Verification items for the finished model (mm, model axes). Face numbers are marked on the shaded views. Coordinates: 2 decimals unless noted, no trailing zeros. Use one line per item in the form item = value. Start each with the question number.
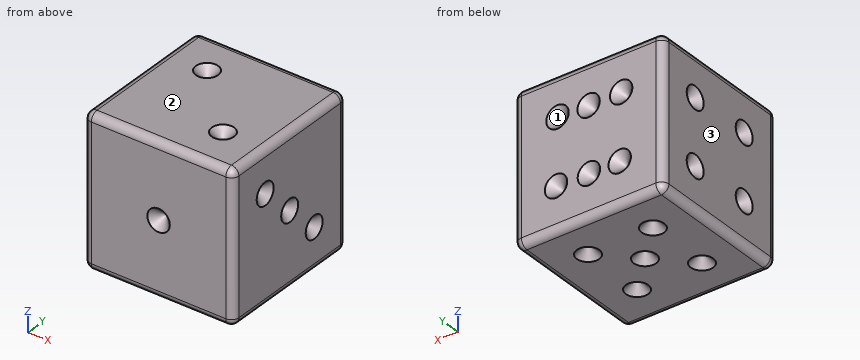
```python
from build123d import *

# Parameters (mm, degrees)
F0_W      = 20
F0_H      = 20
F1_DEPTH  = 20
F2_R      = 1.5
F3_DEPTH  = 1.5
F4_R      = 1
F5_R      = 1.5
F6_DEPTH  = 1.5
F7_R      = 1.5
F8_DEPTH  = 1.5
F9_R      = 1.5
F10_DEPTH = 1.5
F11_R     = 1.5
F12_DEPTH = 1.5
F13_R     = 1.5
F14_DEPTH = 1.5
F15_SIZE  = 1.49999


# Not quite as in the source:
# - a fillet or chamfer is up to 0.001 mm smaller than in the source, because OpenCascade refuses the exact size


with BuildPart() as f1:
    # F0 (on Top) → F1 (new body)
    with BuildSketch(Plane.XY):
        with Locations((10, 10)):
            Rectangle(F0_W, F0_H)
    extrude(amount=F1_DEPTH)

    # F2 (on face) → F3 (cut)
    with BuildSketch(Plane.XZ):
        with Locations((10, 10)):
            Circle(F2_R)
    extrude(amount=-F3_DEPTH, mode=Mode.SUBTRACT)

    # F4
    f4_edges = [f1.edges().sort_by_distance(p)[0] for p in [
        (10, 0, 20),
        (20, 10, 20),
        (20, 0, 10),
        (0, 0, 10),
        (10, 0, 0),
        (20, 10, 0),
        (0, 10, 20),
        (10, 20, 20),
        (0, 10, 0),
        (0, 20, 10),
        (20, 20, 10),
        (10, 20, 0),
    ]]
    fillet(f4_edges, radius=F4_R)

    # F5 (on face) → F6 (cut)
    with BuildSketch(Plane.XY.offset(20)):
        with Locations((5.6568542495, 14.3431457505)):
            Circle(F5_R)
        with Locations((14.3431457505, 5.6568542495)):
            Circle(F5_R)
    extrude(amount=-F6_DEPTH, mode=Mode.SUBTRACT)

    # F7 (on face) → F8 (cut)
    with BuildSketch(Plane.YZ.offset(20)):
        with Locations((5.6568542495, 14.3431457505)):
            Circle(F7_R)
        with Locations((10, 10)):
            Circle(F7_R)
        with Locations((14.3431457505, 5.6568542495)):
            Circle(F7_R)
    extrude(amount=-F8_DEPTH, mode=Mode.SUBTRACT)

    # F9 (on face) → F10 (cut)
    with BuildSketch(Plane(origin=(0, 0, 0), x_dir=(0, -1, 0), z_dir=(-1, 0, 0))):
        with Locations((-14.3431457505, 14.3431457505)):
            Circle(F9_R)
        with Locations((-5.6568542495, 14.3431457505)):
            Circle(F9_R)
        with Locations((-14.3431457505, 5.6568542495)):
            Circle(F9_R)
        with Locations((-5.6568542495, 5.6568542495)):
            Circle(F9_R)
    extrude(amount=-F10_DEPTH, mode=Mode.SUBTRACT)

    # F11 (on face) → F12 (cut)
    with BuildSketch(Plane(origin=(0, 0, 0), x_dir=(1, 0, 0), z_dir=(0, 0, -1))):
        with Locations((5.6568542495, -5.6568542495)):
            Circle(F11_R)
        with Locations((10, -10)):
            Circle(F11_R)
        with Locations((14.3431457505, -5.6568542495)):
            Circle(F11_R)
        with Locations((5.6568542495, -14.3431457505)):
            Circle(F11_R)
        with Locations((14.3431457505, -14.3431457505)):
            Circle(F11_R)
    extrude(amount=-F12_DEPTH, mode=Mode.SUBTRACT)

    # F13 (on face) → F14 (cut)
    with BuildSketch(Plane(origin=(0, 20, 0), x_dir=(-1, 0, 0), z_dir=(0, 1, 0))):
        with Locations((-5.6367907673, 14.3558382988)):
            Circle(F13_R)
        with Locations((-10, 14.3431457505)):
            Circle(F13_R)
        with Locations((-14.1635667533, 14.496743679)):
            Circle(F13_R)
        with Locations((-14.3617270514, 5.7898699306)):
            Circle(F13_R)
        with Locations((-9.9599251616, 5.6883007245)):
            Circle(F13_R)
        with Locations((-5.8349510655, 5.6489654817)):
            Circle(F13_R)
    extrude(amount=-F14_DEPTH, mode=Mode.SUBTRACT)

    # F15 (size 1.5 in the source; OpenCascade refuses exactly that, so slightly less here)
    f15_edges = [f1.edges().sort_by_distance(p)[0] for p in [
        (8.5, 1.5, 10),
        (4.156854, 14.343146, 18.5),
        (12.843146, 5.656854, 18.5),
        (18.5, 4.156854, 14.343146),
        (18.5, 8.5, 10),
        (18.5, 12.843146, 5.656854),
        (1.5, 15.843146, 5.656854),
        (1.5, 15.843146, 14.343146),
        (1.5, 7.156854, 14.343146),
        (1.5, 7.156854, 5.656854),
        (4.156854, 5.656854, 1.5),
        (12.843146, 5.656854, 1.5),
        (8.5, 10, 1.5),
        (4.156854, 14.343146, 1.5),
        (12.843146, 14.343146, 1.5),
        (7.136791, 18.5, 14.355838),
        (11.5, 18.5, 14.343146),
        (15.663567, 18.5, 14.496744),
        (15.861727, 18.5, 5.78987),
        (11.459925, 18.5, 5.688301),
        (7.334951, 18.5, 5.648965),
    ]]
    chamfer(f15_edges, length=F15_SIZE)


solid = f1.part
```
1. Release check for a two-part mould opening along Z. For the marked faces 1, 2 and 3 record: pulls with the +Z half, pulls with the -Z half, needs draft (parallel to the pull), parting line crosses it, or undercut.
2. Material ranges on line 1 along Z through (x, y) = (10.5, 10); line 2 along Z through (x, y) = (15.25, 13.75); line 3 along Y through (x, z) = (14.5, 13.5), recorded low to high.
3. Depth check by flat-ended pin: P1, Ø2.5, axis at x = 14.34, y = 14.34, coming from the -Z side; P2, Ø2.5, axis at x = 5.83, z = 5.65, coming from the +Y side; P3, Ø2.5, axis at x = 14.34, y = 5.66, coming from the +Z side. Enter the tip coordinate at first touch or a pass-through.
Final values:
q1.face_1 = undercut
q1.face_2 = pulls with the +Z half
q1.face_3 = needs draft
q2.line_1 = 1 to 20
q2.line_2 = 0.42 to 20
q2.line_3 = 0 to 19.55
q3.P1 = 0.25
q3.P2 = 19.76
q3.P3 = 19.75
